```python
from build123d import *

# Parameters (mm, degrees)
EXTRUDE_1_DEPTH     = 2
SKETCH_4_R          = 25.034791669
EXTRUDE_2_DEPTH     = 9
SKETCH_5_R          = 1.739871364
SKETCH_7_R          = 3.716982855
EXTRUDE_3_DEPTH     = 6
CHAMFER_1_SIZE      = 0.2
SKETCH_9_R          = 25
CUT_EXTRUDE_2_DEPTH = 0.36
EXTRUDE_4_DEPTH     = 2
SKETCH_13_R         = 4
CUT_EXTRUDE_3_DEPTH = 35


with BuildPart() as part:
    # 草图1 → 凸台-拉伸1 (new body)
    with BuildSketch(Plane.XY):
        with BuildLine():
            Line((40.5, -31.5), (-40.5, -31.5))
            ThreePointArc((-40.5, -31.5), (-44.742640687, -29.742640687), (-46.5, -25.5))
            Line((-46.5, -25.5), (-46.5, 25.5))
            ThreePointArc((-46.5, 25.5), (-44.742640687, 29.742640687), (-40.5, 31.5))
            Line((-40.5, 31.5), (40.5, 31.5))
            ThreePointArc((40.5, 31.5), (44.742640687, 29.742640687), (46.5, 25.5))
            Line((46.5, 25.5), (46.5, -25.5))
            ThreePointArc((46.5, -25.5), (44.742640687, -29.742640687), (40.5, -31.5))
        make_face()
        with BuildLine():
            Line((-43.156854249, 22.5), (-37.5, 28.156854249))
            ThreePointArc((-37.5, 28.156854249), (-31.843145751, 28.156854249), (-31.843145751, 22.5))
            Line((-31.843145751, 22.5), (-37.5, 16.843145751))
            ThreePointArc((-37.5, 16.843145751), (-43.156854249, 16.843145751), (-43.156854249, 22.5))
        make_face(mode=Mode.SUBTRACT)
        with BuildLine():
            Line((37.5, 28.156854249), (43.156854249, 22.5))
            ThreePointArc((43.156854249, 22.5), (43.156854249, 16.843145751), (37.5, 16.843145751))
            Line((37.5, 16.843145751), (31.843145751, 22.5))
            ThreePointArc((31.843145751, 22.5), (31.843145751, 28.156854249), (37.5, 28.156854249))
        make_face(mode=Mode.SUBTRACT)
        with BuildLine():
            Line((31.843145751, -22.5), (37.5, -16.843145751))
            ThreePointArc((37.5, -16.843145751), (43.156854249, -16.843145751), (43.156854249, -22.5))
            Line((43.156854249, -22.5), (37.5, -28.156854249))
            ThreePointArc((37.5, -28.156854249), (31.843145751, -28.156854249), (31.843145751, -22.5))
        make_face(mode=Mode.SUBTRACT)
        with BuildLine():
            Line((-37.5, -28.156854249), (-43.156854249, -22.5))
            ThreePointArc((-43.156854249, -22.5), (-43.156854249, -16.843145751), (-37.5, -16.843145751))
            Line((-37.5, -16.843145751), (-31.843145751, -22.5))
            ThreePointArc((-31.843145751, -22.5), (-31.843145751, -28.156854249), (-37.5, -28.156854249))
        make_face(mode=Mode.SUBTRACT)
    extrude(amount=-EXTRUDE_1_DEPTH)

    # 草图4 → 凸台-拉伸2 (add)
    with BuildSketch(Plane.XY):
        Circle(SKETCH_4_R)
    extrude(amount=EXTRUDE_2_DEPTH)

    # 草图5 → 旋转2 (revolve)
    with BuildSketch(Plane(origin=(0, 0, 0), x_dir=(1, 0, 0), z_dir=(0, 1, 0))):
        with Locations((-25.034791669, -7.260128636)):
            Circle(SKETCH_5_R)
    revolve(axis=Axis((0, 0, 0), (0, 0, 1)))

    # 草图7 → 凸台-拉伸3 (add)
    with BuildSketch(Plane.XY.offset(9)):
        Circle(SKETCH_7_R)
    extrude(amount=EXTRUDE_3_DEPTH)

    # 倒角1
    chamfer_1_edges = [part.edges().sort_by_distance(p)[0] for p in [
        (-3.716982855, 0, 15),
    ]]
    chamfer(chamfer_1_edges, length=CHAMFER_1_SIZE)

    # 草图9 → 切除-拉伸2 (cut)
    with BuildSketch(Plane(origin=(0, 0, -2), x_dir=(-1, 0, 0), z_dir=(0, 0, -1))):
        Circle(SKETCH_9_R)
    extrude(amount=-CUT_EXTRUDE_2_DEPTH, mode=Mode.SUBTRACT)

    # 草图12 → 凸台-拉伸4 (add)
    with BuildSketch(Plane(origin=(0, 0, -2), x_dir=(-1, 0, 0), z_dir=(0, 0, -1))):
        with BuildLine():
            Line((37.5, 28.156854249), (43.156854249, 22.5))
            ThreePointArc((43.156854249, 22.5), (43.156854249, 16.843145751), (37.5, 16.843145751))
            Line((37.5, 16.843145751), (31.843145751, 22.5))
            ThreePointArc((31.843145751, 22.5), (31.843145751, 28.156854249), (37.5, 28.156854249))
        make_face()
        with BuildLine():
            Line((43.156854249, -22.5), (37.5, -28.156854249))
            ThreePointArc((37.5, -28.156854249), (31.843145751, -28.156854249), (31.843145751, -22.5))
            Line((31.843145751, -22.5), (37.5, -16.843145751))
            ThreePointArc((37.5, -16.843145751), (43.156854249, -16.843145751), (43.156854249, -22.5))
        make_face()
        with BuildLine():
            Line((-37.5, -28.156854249), (-43.156854249, -22.5))
            ThreePointArc((-43.156854249, -22.5), (-43.156854249, -16.843145751), (-37.5, -16.843145751))
            Line((-37.5, -16.843145751), (-31.843145751, -22.5))
            ThreePointArc((-31.843145751, -22.5), (-31.843145751, -28.156854249), (-37.5, -28.156854249))
        make_face()
        with BuildLine():
            Line((-43.156854249, 22.5), (-37.5, 28.156854249))
            ThreePointArc((-37.5, 28.156854249), (-31.843145751, 28.156854249), (-31.843145751, 22.5))
            Line((-31.843145751, 22.5), (-37.5, 16.843145751))
            ThreePointArc((-37.5, 16.843145751), (-43.156854249, 16.843145751), (-43.156854249, 22.5))
        make_face()
    extrude(amount=-EXTRUDE_4_DEPTH)

    # 草图13 → 切除-拉伸3 (cut)
    with BuildSketch(Plane(origin=(0, 0, -2), x_dir=(-1, 0, 0), z_dir=(0, 0, -1))):
        with Locations((-37.5, 22.5)):
            Circle(SKETCH_13_R)
        with Locations((-37.5, -22.5)):
            Circle(SKETCH_13_R)
        with Locations((37.5, -22.5)):
            Circle(SKETCH_13_R)
        with Locations((37.5, 22.5)):
            Circle(SKETCH_13_R)
    extrude(amount=-CUT_EXTRUDE_3_DEPTH, mode=Mode.SUBTRACT)


solid = part.part
```
Design review of the part built by this model. Coordinates are the model's own, in mm. A direction names the side the tool comes from. Give positions to 0.01 mm unless a question says otherwise; leave off trailing zeros. Order: outer loops, then holes, each group sorted by start corner. A loop starts at its lowest first (then second) coordinate and runs counter-clockwise, first axis right, second up. Notation, with made-up numbers: (89.5, 21.5) - (106.5, 21.5) arc R24 ccw to (106.5, 31.5) - close; hole circle Ø4 at (33, -22). An arc over 180 degrees is marked (long way). Use a Markdown table: item, result. Add a question column.
(1) Clearance check with flat-ended pins moving along their axes: P1, Ø1, axis at x = -19.5, z = 7.5, coming from the +Y side; P2, Ø5, axis at x = -19.5, z = 5.5, coming from the -Y side; P3, Ø3, axis at x = -15, y = 5, coming from the +Z side. State where each tip first meets the part, or that it passes through.
(2) Wall thickness on probe 1 along Y at (x, z) = (37.5, -1.4); probe 2 along Z at (x, y) = (22.5, -8.5); probe 3 along Z at (x, y) = (1.5, 27): over which ranges is each line inside the solid? List them lowest first. Write a range as [from, to].
(3) Add section D-D on z = 12.5. Give the boundary of the cut face in (x, y), then the cut area to 3 significant figures.
(4) Machinability: for faces 5 (the face through (-46.5, 0, -1)), 6 (the face through (-2.95, -2.26, 11.86)), 7 (the face through (0, 0, -1.64)), which of the approach directions +Z, -Z, +X, -X, +Y, -Y give a long, thin tool a straight path to every point of the face, cutting with its end or side? Answer none if there is none.
(5) Add section C-C on y = -22.5. Give the number of separate pieces and of enclosed holes in the cut face, then the cut area to 3 significant figures.
(6) Mouldability with a two-part tool opening along Y and no side actions: class faces 1 (the face through (-23.846, 7.509, -1.823)), 2 (the face through (1, -31.5, -1)), 3 (the face through (23.126, -9.588, 2.721)), 4 (the face through (38.021, 26.466, -1.014)) as +Y half, -Y half, draft (parallel to the pull), parting line (faces both ways), or undercut.
(7) Add section B-B on x = 0. Give the boundary of the cut face in (y, z), then the cut area to 3 significant figures.
(8) Add section A-A on x = 37.5. Give the boundary of the cut face in (y, z), then the cut area to 3 significant figures.
Report:
| question | item | result |
|---|---|---|
| 1 | P1 | stops at y = 18.85 |
| 1 | P2 | stops at y = -20.31 |
| 1 | P3 | stops at z = 9 |
| 2 | probe 1 | y = [-31.5, -26.5], [-18.5, 18.5], [26.5, 31.5] |
| 2 | probe 2 | z = [-1.64, 9] |
| 2 | probe 3 | z = [-2, 0] |
| 3 | outline | circle Ø7.43 at (0, 0) |
| 3 | area | 43.4 mm² |
| 4 | face 5 | +Z, -Z, -X, +Y, -Y |
| 4 | face 6 | +Z |
| 4 | face 7 | -Z |
| 5 | separate pieces | 3 |
| 5 | enclosed holes | 0 |
| 5 | area | 363 mm² |
| 6 | face 1 | undercut |
| 6 | face 2 | -Y half |
| 6 | face 3 | parting line |
| 6 | face 4 | undercut |
| 7 | outline | (-31.5, -2) - (-25, -2) - (-25, -1.64) - (25, -1.64) - (25, -2) - (31.5, -2) - (31.5, 0) - (25.03, 0) - (25.03, 5.52) arc R1.74 ccw to (25.03, 9) - (3.72, 9) - (3.72, 14.8) - (3.52, 15) - (-3.52, 15) - (-3.72, 14.8) - (-3.72, 9) - (-25.03, 9) arc R1.74 ccw to (-25.03, 5.52) - (-25.03, 0) - (-31.5, 0) - close |
| 7 | area | 613 mm² |
| 8 | outline | (-31.5, -2) - (-26.5, -2) - (-26.5, 0) - (-31.5, 0) - close; (-18.5, -2) - (18.5, -2) - (18.5, 0) - (-18.5, 0) - close; (26.5, -2) - (31.5, -2) - (31.5, 0) - (26.5, 0) - close |
| 8 | area | 94.0 mm² |
